Can you work these out from the model? Positions are in its coordinate system, mm. A direction names the side the tool comes from. Give positions to 0.01 mm unless a question says otherwise; leave off trailing zeros. Loops run counter-clockwise (first coordinate to the right, second up) from the corner with the lowest first, then second, coordinate; pieces in that order, holes last. Notation, with made-up numbers: M -20.5,-21.75 L 13.5,-21.75 A20 cw 13.5,15.25 Z; hole C 24,32 d5. An arc over 180 degrees is marked long. Put each result on its own line as item: value. Start each with the question number.
1) For faces 1 (the cylindrical face through (-0.36, 0.92, 1.52)), 2 (the cylindrical face through (14.516, 3.252, 6.451)), which set-ups out of +Z, -Z, +X, -X, +Y, -Y let a thin tool reach every point of the face, with its end or its side?
2) Please list where these lines run through material, in increasing order: line 1 along Z through (x, y) = (3, -7.5); line 2 along X through (y, z) = (-13.5, 4.75); line 3 along X through (y, z) = (-10.5, 8). Write a range as from..to.
3) Imagine slicing it at C-C (x = -8). Write out the boundary of the cut face in (y, z).
4) Imagine slicing it at B-B (y = 0). Write out the boundary of the cut face in (x, z).
5) If we mould it in two halves opening along Y, with no side actions, what happens to faces 3 (the flat face through (3, 0, 3)), 4 (the cylindrical face through (-4.336, 19.524, 4.93)), 5 (the flat face through (-3, -15, 10))? For each: +Y half, -Y half, draft (parallel to the pull), parting line (faces both ways), or undercut.
6) Imagine slicing it at A-A (y = -9). Write out the boundary of the cut face in (x, z), then the cut area to 3 significant figures.
7) For P1, Ø2, axis at x = -7.5, z = 3.5, coming from the -Y side; P2, Ø5, axis at y = -7, z = 2, coming from the -X side; P3, Ø6, axis at y = 13, z = 6, coming from the -X side, each with a flat end and sliding along its axis, tell me the tip position at first contact or that it passes through.
8) Imagine slicing it at D-D (z = 2.5). Write out the boundary of the cut face in (x, y).
Autodesk Fusion 360 part; units mm, degrees
sketch "Sketch1" plane through (0, 0, 0) normal (0, 0, 1) x (1, 0, 0)
  circle A0 centre (0, 0) radius 20
extrude "Extrude1" add sketch "Sketch1" along normal blind 10
hole "Hole1" at (-0.1278, 0, 10) direction (0, 0, -1) diameter 30 depth 7 tip angle 180
hole "Hole2" at (-0.0621, -0.0347, 0) direction (0, 0, 1) diameter 2 depth 7 tip angle 180
Recorded:
1. face 1: +Z, -Z
1. face 2: +Z
2. line 1: 0..3
2. line 2: -14.76..-6.67, 6.41..14.76
2. line 3: -17.02..-10.84, 10.58..17.02
3. outline: M -18.33,0 L 18.33,0 L 18.33,10 L 12.77,10 L 12.77,3 L -12.77,3 L -12.77,10 L -18.33,10 Z
4. outline: M -20,0 L -1.06,0 L -1.06,3 L -15.13,3 L -15.13,10 L -20,10 Z; M 0.94,0 L 20,0 L 20,10 L 14.87,10 L 14.87,3 L 0.94,3 Z
5. face 3: undercut
5. face 4: parting line
5. face 5: draft
6. outline: M -17.86,0 L 17.86,0 L 17.86,10 L 11.87,10 L 11.87,3 L -12.13,3 L -12.13,10 L -17.86,10 Z
6. area: 189 mm²
7. P1: y = -18.91
7. P2: x = -19.49
7. P3: x = -17.32
8. outline: C 0,0 d40; hole C -0.06,-0.03 d2
